Read the model definition and answer for the solid it produces. Units are mm, in the model's axes. Face numbers are marked on the shaded views. Give positions to 0.01 mm unless a question says otherwise; leave off trailing zeros. Write each loop counter-clockwise with the first axis right and the second up, starting at its lowest first coordinate (ties: lowest second). Pieces come first, ordered by that corner, then holes. Notation, with made-up numbers: M -14,0.5 L 29,0.5 A15 cw 29,24.5 Z; hole C -18,-1.75 d5. An arc over 180 degrees is marked long. Use a Markdown table: item, result. Add a question column.
Item 1: A cutting plane is placed at A-A on x = 0. Determine the outline of the cut face in (y, z), then the cut area to 3 significant figures.
Item 2: A cutting plane is placed at B-B on y = 11. Determine the outline of the cut face in (x, z), then the cut area to 3 significant figures.
Item 3: The mould has two halves that part along X. Classify the marked faces 1, 2 and 3: pulls with the +X half, pulls with the -X half, needs draft (parallel to the pull), parting line crosses it, or undercut.
Item 4: Given P1, Ø4, axis at y = 14.5, z = 10, coming from the -X side; P2, Ø6, axis at y = 12, z = 19, coming from the -X side; P3, Ø8, axis at x = -28.5, y = 14, coming from the -Z side, each flat-ended and moving along its own axis, determine where each tip first touches the part or whether it passes through.
Item 5: A cutting plane is placed at C-C on x = 30. Determine the outline of the cut face in (y, z), then the cut area to 3 significant figures.
Item 6: Consider probe 1 along Z at (x, y) = (0, 12.25); probe 2 along X at (y, z) = (16.5, 0); probe 3 along Y at (x, z) = (-33.5, 11). Determine where each line is inside the solid, lowest interval first. Write a range as [from, to].
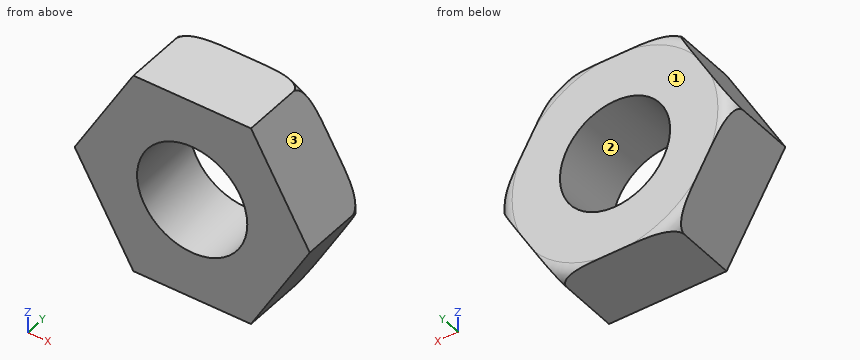
from build123d import *

# Parameters (mm, degrees)
BOSS_EXTRUDE1_DEPTH = 25
SKETCH3_R           = 18.75
CUT_EXTRUDE1_DEPTH  = 49


with BuildPart() as part:
    # Sketch1 → Boss-Extrude1 (new body)
    with BuildSketch(Plane(origin=(0, 0, 0), x_dir=(1, 0, 0), z_dir=(0, 1, 0))):
        Polygon((40, 0), (20, 34.641016151), (-20, 34.641016151), (-40, 0), (-20, -34.641016151), (20, -34.641016151), align=None)
    extrude(amount=BOSS_EXTRUDE1_DEPTH)

    # Sketch2 → Cut-Revolve1 (revolve, cut)
    with BuildSketch(Plane.XY):
        with BuildLine():
            Line((-40, 19.787670443), (-40, 20))
            ThreePointArc((-40, 20), (-38.535533906, 23.535533906), (-35, 25))
            Line((-35, 25), (-37.757743641, 31.268029575))
            Line((-37.757743641, 31.268029575), (-44.972742857, 23.763902868))
            Line((-44.972742857, 23.763902868), (-40, 19.787670443))
        make_face()
    revolve(axis=Axis((0, 25, 0), (0, 1, 0)), mode=Mode.SUBTRACT)

    # Sketch3 → Cut-Extrude1 (cut)
    with BuildSketch(Plane(origin=(0, 25, 0), x_dir=(1, 0, 0), z_dir=(0, 1, 0))):
        Circle(SKETCH3_R)
    extrude(amount=-CUT_EXTRUDE1_DEPTH, mode=Mode.SUBTRACT)


solid = part.part
Filled in:
| question | item | result |
|---|---|---|
| 1 | outline | M 0,-34.64 L 25,-34.64 L 25,-18.75 L 0,-18.75 Z; M 0,18.75 L 25,18.75 L 25,34.64 L 0,34.64 Z |
| 1 | area | 795 mm² |
| 2 | outline | M -40,0 L -20,-34.64 L 20,-34.64 L 40,0 L 20,34.64 L -20,34.64 Z; hole C 0,0 d37.5 |
| 2 | area | 3,050 mm² |
| 3 | face 1 | needs draft |
| 3 | face 2 | undercut |
| 3 | face 3 | pulls with the +X half |
| 4 | P1 | x = -35.38 |
| 4 | P2 | x = -30.76 |
| 4 | P3 | z = -26.85 |
| 5 | outline | M 0,-17.32 L 25,-17.32 L 25,17.32 L 0,17.32 Z |
| 5 | area | 866 mm² |
| 6 | probe 1 | [-34.64, -18.75], [18.75, 34.64] |
| 6 | probe 2 | [-40, -18.75], [18.75, 40] |
| 6 | probe 3 | [0, 24.99] |
